Verification items for the finished model (mm, model axes). A direction names the side the tool comes from. Round coordinates to 2 decimals unless told otherwise and drop trailing zeros. Loops run counter-clockwise (first coordinate to the right, second up) from the corner with the lowest first, then second, coordinate; pieces in that order, holes last. Notation, with made-up numbers: (17, 49) -> (73, 49) arc R24 ccw to (73, 61) -> close; hole circle Ø10 at (41.25, 70). An arc over 180 degrees is marked (long way). Use CSV: the item, a comma, the result in double quotes. Start each with the question number.
Autodesk Inventor part; units mm, degrees
ref_plane "Work Plane1" through (-20.5163, 50.8, -469.9) normal (1, 0, 0) x (0, 0, -1)
ref_plane "YZ Plane" through (0, 0, 0) normal (1, 0, 0) x (0, 1, 0)
ref_plane "XZ Plane" through (0, 0, 0) normal (0, 1, 0) x (-1, 0, 0)
sketch "Sketch1" plane through (0, 0, 0) normal (0, 1, 0) x (-1, 0, 0)
  line L0 (0, 0) -> (0, -469.9)
  line L1 (0, -469.9) -> (0, -122.0086)
  line L2 (0, -469.9) -> (20.5163, -469.9)
  line L3 (20.5163, -469.9) -> (0, 0)
  dimension "d0" = 469.9
  dimension "d1" = 2.5
extrude "Extrusion1" add sketch "Sketch1" along normal blind 50.8
ref_plane "Work Plane1" through (-20.5163, 50.8, -469.9) normal (1, 0, 0) x (0, 0, -1)
sketch "Sketch2" plane through (0, 0, 0) normal (1, 0, 0) x (0, 0, -1)
  line L0 (0, 0) -> (469.9, 0)
  line L1 (0, 50.8) -> (469.9, 50.8)
  line L2 (0, 0) -> (469.9, 0)
  line L3 (469.9, 0) -> (469.9, 50.8)
  line L4 (469.9, 50.8) -> (0, 50.8)
  line L5 (0, 50.8) -> (0, 0)
extrude "Extrusion2" add sketch "Sketch2" along normal blind 12.7
sketch "Sketch4" plane through (-20.5163, 50.8, -469.9) normal (1, 0, 0) x (0, 0, -1)
  line L0 (0, -50.8) -> (0, 0) construction
  line L1 (0, -25.4) -> (-279.4, -25.4) construction
  line L2 (0, -50.8) -> (-469.9, -50.8) construction
  line L3 (-469.9, -50.8) -> (-469.9, 0) construction
  point P0 (-381, -25.4)
  point P1 (-123.825, -25.4)
  point P2 (-469.9, 0)
  dimension "d16" = 25.4
  dimension "d17" = 88.9
  dimension "d18" = 346.075
hole "Hole2" at (-20.5163, 25.4, -88.9) at (-20.5163, 25.4, -346.075) direction (1, 0, 0) diameter 6.7564 end through all
sketch "Sketch6" plane through (-20.5163, 50.8, -469.9) normal (1, 0, 0) x (0, 0, -1)
  circle A0 centre (-123.825, -25.4) radius 3.3782
  line L0 (-130.2408, -25.4) -> (-127.0329, -19.8438)
  line L1 (-127.0329, -19.8438) -> (-120.6171, -19.8438)
  line L2 (-120.6171, -19.8438) -> (-117.4092, -25.4)
  line L3 (-117.4092, -25.4) -> (-120.6171, -30.9563)
  line L4 (-120.6171, -30.9563) -> (-127.0329, -30.9562)
  line L5 (-127.0329, -30.9562) -> (-130.2408, -25.4)
  circle A1 centre (-381, -25.4) radius 3.3782
  line L6 (-387.4158, -25.4) -> (-384.2079, -19.8438)
  line L7 (-384.2079, -19.8438) -> (-377.7921, -19.8438)
  line L8 (-377.7921, -19.8438) -> (-374.5842, -25.4)
  line L9 (-374.5842, -25.4) -> (-377.7921, -30.9563)
  line L10 (-377.7921, -30.9563) -> (-384.2079, -30.9563)
  line L11 (-384.2079, -30.9563) -> (-387.4158, -25.4)
  line L12 (0, 0) -> (-469.9, 0)
  point P0 (-469.9, -50.8)
  dimension "d26" = 11.1125
extrude "Extrusion3" cut sketch "Sketch6" along normal blind 23.368
ref_plane "Work Plane2" through (-20.5163, 0, -234.95) normal (0, 0, -1) x (-1, 0, 0)
split "Split2" plane through (-20.5163, 0, -234.95) removes the side toward (0, 0, -1)
sketch "Sketch7" plane through (-20.5163, 50.8, -469.9) normal (1, 0, 0) x (0, 0, -1)
  line L0 (-120.65, -38.1) -> (-349.25, -38.1)
  line L1 (-349.25, -38.1) -> (-349.25, -12.7)
  line L2 (-349.25, -12.7) -> (-120.65, -12.7)
  line L3 (-120.65, -12.7) -> (-120.65, -38.1)
  line L4 (-234.95, -50.8) -> (-234.95, 0)
  line L5 (-120.65, -38.1) -> (-349.25, -12.7) construction
  line L6 (-349.25, -38.1) -> (-120.65, -12.7) construction
  point P0 (-469.9, -50.8)
  point P1 (-234.95, -25.4)
  dimension "d30" = 25.4
  dimension "d31" = 228.6
extrude "Extrusion4" cut sketch "Sketch7" along normal through all
equation "\"d0\" = lengthOfFixture"
equation "\"d1\" = cutAngle"
equation "\"d2\" = heightOfJig"
equation "\"d4\" = addedDepthToSupportBolts"
equation "\"d16\" = heightOfBoltHolt"
equation "\"d26\" = hexBoltDiameter"
equation "\"d27\" = depthOfHoleForHexBolt + clearanceForHexbolt"
equation "\"lengthOfFixture\" = 469.9"
equation "\"cutAngle\" = 2.5deg"
equation "\"bottomToFirstHole\" = 88.9"
equation "\"distanceBetweenBolts\" = 257.175"
equation "\"bottomToSecondHole\" = bottomToFirstHole + distanceBetweenBolts"
equation "\"heightOfBoltHolt\" = 25.4"
equation "\"boltSize\" = 6.35"
equation "\"heightOfJig\" = 50.8"
equation "\"addedDepthToSupportBolts\" = 12.7"
equation "\"depthOfHoleForHexBolt\" = 22.86"
equation "\"hexBoltDiameter\" = 11.1125"
equation "\"clearanceForHexbolt\" = 0.508"
equation "\"d29\" = -0.5 * lengthOfFixture"
properties part number "jigForRipCutsA" material "PC/ABS Plastic"
Q1. Thickness scan on L1, parallel to Y at x = 11.25, z = -182; L2, parallel to Y at x = 0, z = -89; L3, parallel to Z at x = 8.75, y = 25.4. Record the ranges inside material, lowest first. Write a range as from..to.
Q2. Depth check by flat-ended pin: pin 1 Ø10 at (y, z) = (9.5, -114.5) entering from -X; pin 2 Ø9 at (y, z) = (24, -92) entering from -X. Enter the tip coordinate at first touch or a pass-through.
Q3. Cross-section at A-A (z = -88.9). Record the boundary of the cut face in (x, y).
Q4. Cross-section at D-D (z = -171). Record the boundary of the cut face in (x, y).
Q5. Cross-section at C-C (z = -133). Record the boundary of the cut face in (x, y).
Q6. Tool access check on faces 4 (the face through (2.852, 28, -92)), 5 (the face through (1, 12.7, -179)), 6 (the face through (7.845, 25.251, -92.275)). Record the directions out of +Z, -Z, +X, -X, +Y, -Y that give a thin tool (end or side, any length) a straight path to the whole face; none if there is none.
Q7. Cross-section at B-B (y = 46). Record the boundary of the cut face in (x, z).
Q8. Release check for a two-part mould opening along Z. For faces 1 (the face through (-0.5, 22.6, -84.1)), 2 (the face through (6, 26, 0)), 3 (the face through (4, 50.8, -116)) record: +Z half, -Z half, draft (parallel to the pull), parting line (faces both ways), or undercut.
Answer list:
1,L1,"y = 0..12.7, 38.1..50.8"
1,L2,"y = 0..19.84, 30.96..50.8"
1,L3,"z = -120.65..-92.28, -85.52..0"
2,pin 1,"stops at x = -5.22"
2,pin 2,"stops at x = -4.21"
3,outline,"(-3.88, 0) -> (12.7, 0) -> (12.7, 22.02) -> (2.85, 22.02) -> (2.85, 19.84) -> (-3.88, 19.84) -> close; (-3.88, 30.96) -> (2.85, 30.96) -> (2.85, 28.78) -> (12.7, 28.78) -> (12.7, 50.8) -> (-3.88, 50.8) -> close"
4,outline,"(-7.47, 0) -> (12.7, 0) -> (12.7, 12.7) -> (-7.47, 12.7) -> close; (-7.47, 38.1) -> (12.7, 38.1) -> (12.7, 50.8) -> (-7.47, 50.8) -> close"
5,outline,"(-5.81, 0) -> (12.7, 0) -> (12.7, 12.7) -> (-5.81, 12.7) -> close; (-5.81, 38.1) -> (12.7, 38.1) -> (12.7, 50.8) -> (-5.81, 50.8) -> close"
6,face 4,"-X"
6,face 5,"-Z, +X, -X"
6,face 6,"+X, -X"
7,outline,"(-10.26, -234.95) -> (12.7, -234.95) -> (12.7, 0) -> (0, 0) -> close"
8,face 1,"undercut"
8,face 2,"+Z half"
8,face 3,"draft"
